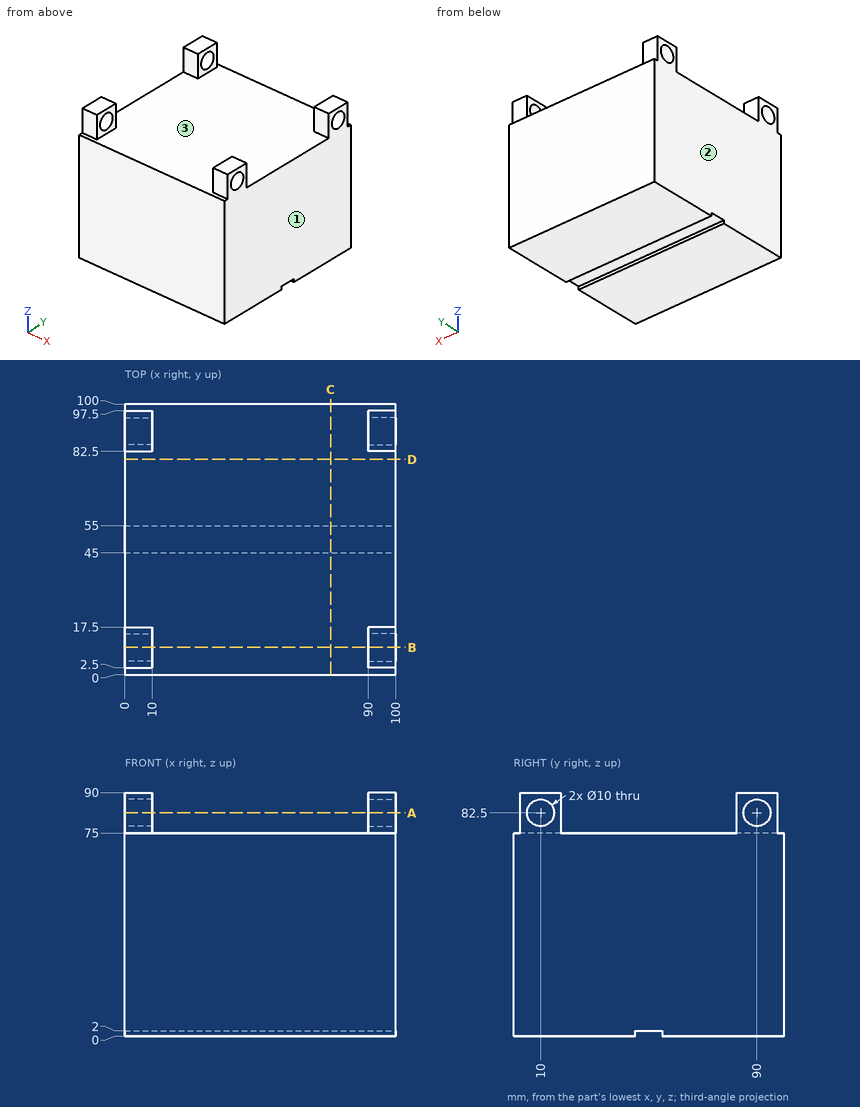
Job drawing, mm, ordinate dimensions from the low corner. One solid piece. Coordinates: 2 decimals unless noted, no trailing zeros. Write each loop counter-clockwise with the first axis right and the second up, starting at its lowest first coordinate (ties: lowest second). Pieces come first, ordered by that corner, then holes. Notation, with made-up numbers: (-4, 58) - (27, 58) arc R16 ccw to (27, 70) - close; hole circle Ø6 at (47, 73.5). An arc over 180 degrees is marked (long way). Use a Markdown table: item, result. Add a question column.
Item 1: Mould opens along X. For the marked faces 1, 2 and 3 say: pulls with the +X half, pulls with the -X half, needs draft (parallel to the pull), parting line crosses it, or undercut.
Item 2: Drill centre lines: L1, parallel to Z at x = 96, y = 90; L2, parallel to Y at x = 92.5, z = 82.5; L3, parallel to Z at x = 12.5, y = 8.5. Where is each one in solid material? Low to high. Write a range as from..to.
Item 3: Band-saw the part on B-B, the plane y = 10. Give the cut face in (x, z).
Item 4: Flat gauge pins, fed straight in: pin 1 (1.6 mm diameter, centred on x = 31, z = 1.5, fed in from -Y); pin 2 (8 mm diameter, centred on x = 95.5, z = 85, fed in from +Y); pin 3 (4.5 mm diameter, centred on y = 9, z = 82.5, fed in from -X); pin 4 (3 mm diameter, centred on x = 7.5, z = 79.5, fed in from -Y). Where does each tip first touch, or does it go through?
Item 5: Band-saw the part on D-D, the plane y = 79.5. Give the cut face in (x, z).
Item 6: Band-saw the part on A-A, the plane z = 82.5. Give the number of separate pieces and of enclosed holes in the cut face, and give its area (3 significant figures).
Item 7: Band-saw the part on C-C, the plane x = 76. Give the cut face in (y, z), and give its area (3 significant figures).
Numbers:
| question | item | result |
|---|---|---|
| 1 | face 1 | pulls with the +X half |
| 1 | face 2 | pulls with the -X half |
| 1 | face 3 | undercut |
| 2 | L1 | 0..77.5, 87.5..90 |
| 2 | L2 | 2.5..5, 15..17.5, 82.5..85, 95..97.5 |
| 2 | L3 | 0..75 |
| 3 | outline | (0, 0) - (100, 0) - (100, 77.5) - (90, 77.5) - (90, 75) - (10, 75) - (10, 77.5) - (0, 77.5) - close; (0, 87.5) - (10, 87.5) - (10, 90) - (0, 90) - close; (90, 87.5) - (100, 87.5) - (100, 90) - (90, 90) - close |
| 4 | pin 1 | y = 0 |
| 4 | pin 2 | y = 97.5 |
| 4 | pin 3 | through |
| 4 | pin 4 | y = 2.5 |
| 5 | outline | (0, 0) - (100, 0) - (100, 75) - (0, 75) - close |
| 6 | separate pieces | 8 |
| 6 | enclosed holes | 0 |
| 6 | area | 200 mm2 |
| 7 | outline | (0, 0) - (45, 0) - (45, 2) - (55, 2) - (55, 0) - (100, 0) - (100, 75) - (0, 75) - close |
| 7 | area | 7,480 mm2 |
